Autodesk Inventor part; units mm, degrees
sketch "Sketch1" plane through (0, 0, 0) normal (0, 1, 0) x (-1, 0, 0)
  circle A0 centre (0, 0) radius 68.75
  dimension "d0" = 137.5
extrude "Extrusion1" add sketch "Sketch1" along normal blind 27.5
sketch "Sketch2" plane through (0, 27.5, 0) normal (0, 1, 0) x (1, 0, 0)
  circle A0 centre (0, 0) radius 66
  dimension "d4" = 132
extrude "Extrusion2" cut sketch "Sketch2" against normal blind 22.5
sketch "Sketch3" plane through (0, 5, 0) normal (0, 1, 0) x (1, 0, 0)
  circle A0 centre (0, 0) radius 68.75
  line L0 (0, 68.75) -> (0, 41.75)
  arc A1 (7.1286, 29.4112) -> (-7.3714, 29.5547) centre (0, 41.75) ccw
  line L1 (8.5358, 25.4622) -> (-8.9642, 25.4622)
  line L2 (8.5358, 25.4622) -> (8.5358, 28.5136)
  line L3 (-8.9642, 25.4622) -> (-8.9642, 28.7999)
  line L4 (-7.3714, 29.5547) -> (-7.3714, 27.0547)
  line L5 (-7.3714, 27.0547) -> (7.1286, 27.0547)
  line L6 (7.1286, 27.0547) -> (7.1286, 29.4112)
  arc A2 (19.25, 38.25) -> (19.25, 45.25) centre (19.25, 41.75) ccw
  line L7 (19.25, 45.25) -> (15.3562, 45.25)
  line L8 (19.25, 38.25) -> (15.3562, 38.25)
  arc A3 (-19.25, 45.25) -> (-19.25, 38.25) centre (-19.25, 41.75) ccw
  line L9 (-19.25, 45.25) -> (-15.3562, 45.25)
  line L10 (-19.25, 38.25) -> (-15.3562, 38.25)
  arc A4 (-15.3562, 38.25) -> (-8.9642, 28.7999) centre (0, 41.75) ccw
  arc A5 (8.5358, 28.5136) -> (15.3562, 38.25) centre (0, 41.75) ccw
  arc A6 (15.3562, 45.25) -> (-15.3562, 45.25) centre (0, 41.75) ccw
  dimension "d7" = 27
  dimension "d8" = 28.5
  dimension "d12" = 17.5
  dimension "d14" = 2.5
  dimension "d15" = 14.5
extrude "Extrusion3" add sketch "Sketch3" along normal blind 19.5 contours A6 L7 A2 L8 A5 L2 L1 L3 A4 L10 A3 L9
sketch "Sketch4" plane through (0, 24.5, 0) normal (0, 1, 0) x (1, 0, 0)
  line L0 (-8.9642, 25.4622) -> (8.5358, 25.4622)
  line L1 (-0.002, 25.4622) -> (2.998, 25.4622)
  line L2 (2.998, 25.4622) -> (2.998, 27.0547)
  line L3 (2.998, 27.0547) -> (-3.002, 27.0547)
  line L4 (7.1286, 27.0547) -> (-7.3714, 27.0547)
  line L5 (-3.002, 27.0547) -> (-3.002, 25.4622)
  line L6 (-3.002, 25.4622) -> (-0.002, 25.4622)
  point P0 (0, 0)
  dimension "d18" = 3
  dimension "d19" = 6
extrude "Extrusion4" cut sketch "Sketch4" against normal blind 4
sketch "Sketch5" plane through (0, 24.5, 0) normal (0, 1, 0) x (1, 0, 0)
  arc A0 (-19.25, 45.25) -> (-19.25, 38.25) centre (-19.25, 41.75) ccw
  circle A1 centre (-19.25, 41.75) radius 2
  arc A2 (19.25, 38.25) -> (19.25, 45.25) centre (19.25, 41.75) ccw
  circle A3 centre (19.25, 41.75) radius 2
  point P0 (0, 0)
  dimension "d24" = 4
  dimension "d25" = 4
extrude "Extrusion5" cut sketch "Sketch5" against normal blind 19
sketch "Sketch6" plane through (0, 5, 0) normal (0, 1, 0) x (1, 0, 0)
  line L0 (-30, 0) -> (-30, 17.25)
  line L1 (-30, 17.25) -> (-62, 17.25)
  line L2 (-62, 17.25) -> (-62, -17.25)
  line L3 (-62, -17.25) -> (-30, -17.25)
  line L4 (-30, -17.25) -> (-30, 0)
  point P0 (0, 0)
  dimension "d28" = 30
  dimension "d29" = 17.25
  dimension "d30" = 32
  dimension "d31" = 90
  dimension "d32" = 34.5
extrude "Extrusion6" cut sketch "Sketch6" against normal blind 2.75
sketch "Sketch7" plane through (0, 5, 0) normal (0, 1, 0) x (1, 0, 0)
  line L0 (-30, 17.25) -> (-30, -17.25)
  line L1 (-30, 0) -> (-26.25, 0)
  line L2 (-26.25, 0) -> (-26.25, 10.5)
  line L3 (-26.25, 10.5) -> (-26.25, -10.5) construction
  line L4 (-22.5, 6.75) -> (-22.5, -6.75)
  line L5 (-30, -6.75) -> (-30, 6.75)
  arc A0 (-22.5, 6.75) -> (-30, 6.75) centre (-26.25, 6.75) ccw
  arc A1 (-30, -6.75) -> (-22.5, -6.75) centre (-26.25, -6.75) ccw
  line L6 (-26.25, 0) -> (36.25, 0)
  line L7 (36.25, 0) -> (36.25, 10.5)
  line L8 (36.25, 10.5) -> (36.25, -10.5) construction
  line L9 (32.5, 6.75) -> (32.5, -6.75)
  line L10 (40, -6.75) -> (40, 6.75)
  arc A2 (40, 6.75) -> (32.5, 6.75) centre (36.25, 6.75) ccw
  arc A3 (32.5, -6.75) -> (40, -6.75) centre (36.25, -6.75) ccw
  line L11 (36.25, 10.5) -> (57.25, 10.5) construction
  point P0 (0, 0)
  dimension "d36" = 3.75
  dimension "d37" = 10.5
  dimension "d38" = 21
  dimension "d39" = 62.5
  dimension "d40" = 10.5
  dimension "d41" = 21
  dimension "d42" = 90
  dimension "d43" = 7.5
extrude "Extrusion7" add sketch "Sketch7" along normal blind 18
sketch "Sketch8" plane through (0, 5, 0) normal (0, 1, 0) x (1, 0, 0)
  line L0 (-22.5, 6.75) -> (-22.5, -6.75)
  line L1 (-22.5, 0) -> (-22.5, 10.5)
  line L2 (-22.5, 10.5) -> (31.5, 10.5)
  line L3 (31.5, 10.5) -> (31.5, -58.1)
  line L4 (31.5, -58.1) -> (-22.5, -58.1)
  line L5 (-22.5, -58.1) -> (-22.5, 10.5)
  point P0 (0, 0)
  dimension "d46" = 10.5
  dimension "d47" = 54
  dimension "d48" = 68.6
extrude "Extrusion8" cut sketch "Sketch8" against normal blind 3
ref_plane "Work Plane1" through (-22.5, 2, 58.1) normal (0, 0, -1) x (-1, 0, 0)
sketch "Sketch9" plane through (-22.5, 2, 58.1) normal (0, 0, -1) x (-1, 0, 0)
  line L0 (-53.8112, 3) -> (0, 3)
  line L1 (0, 3) -> (-9, 3)
  line L2 (-9, 3) -> (-9, 15)
  line L3 (-9, 15) -> (-21.5, 15)
  line L4 (-21.5, 15) -> (-21.5, 3)
  line L5 (-21.5, 3) -> (-9, 3)
  line L6 (-54, 0) -> (0, 0)
  point P0 (-22.5, -2)
  dimension "d52" = 12
  dimension "d53" = 12.5
extrude "Extrusion9" cut sketch "Sketch9" against normal blind 102
ref_plane "Work Plane2" through (68.75, 0, 0) normal (1, 0, 0) x (0, 1, 0)
sketch "Sketch10" plane through (68.75, 0, 0) normal (1, 0, 0) x (0, 1, 0)
  line L0 (0, -68.75) -> (0, 68.75)
  line L1 (0, 0) -> (2, 0)
  line L2 (1.5818, 0) -> (1.5818, -10)
  line L3 (1.5818, -10) -> (21.5818, -10)
  line L4 (21.5818, -10) -> (21.5818, 10)
  line L5 (5, 10.5) -> (23, 10.5)
  line L6 (21.5818, 10) -> (1.5818, 10)
  line L7 (1.5818, 10) -> (1.5818, 0)
  line L8 (2, -10.5) -> (2, 58.1)
  point P0 (2, 10)
  point P1 (2, -10)
  dimension "d64" = 10
  dimension "d65" = 20
  dimension "d66" = 20
  dimension "d67" = 20
extrude "Extrusion10" cut sketch "Sketch10" against normal blind 5 contours L8 L6 L4 L3
sketch "Sketch11" plane through (0, 23, 0) normal (0, 1, 0) x (1, 0, 0)
  arc A0 (40, 6.75) -> (32.5, 6.75) centre (36.25, 6.75) ccw
  circle A1 centre (36.25, 6.75) radius 2
  arc A2 (32.5, -6.75) -> (40, -6.75) centre (36.25, -6.75) ccw
  circle A3 centre (36.25, -6.75) radius 2
  arc A4 (-22.5, 6.75) -> (-30, 6.75) centre (-26.25, 6.75) ccw
  circle A5 centre (-26.25, 6.75) radius 2
  arc A6 (-30, -6.75) -> (-22.5, -6.75) centre (-26.25, -6.75) ccw
  circle A7 centre (-26.25, -6.75) radius 2
  point P0 (0, 0)
  dimension "d70" = 4
  dimension "d71" = 4
  dimension "d72" = 4
  dimension "d73" = 4
extrude "Extrusion11" cut sketch "Sketch11" against normal blind 12
properties part number "gehäuse_scan"
Geometry check sheet. Reference: the model listing, model coordinates, mm. A direction names the side the tool comes from. Give positions to 0.01 mm unless a question says otherwise; leave off trailing zeros. Loops run counter-clockwise (first coordinate to the right, second up) from the corner with the lowest first, then second, coordinate; pieces in that order, holes last. Notation, with made-up numbers: (57.25, 72.5) - (85.25, 72.5) arc R21 ccw to (85.25, 95.5) - close; hole circle Ø10 at (66.25, -1). An arc over 180 degrees is marked (long way). Use CSV: the item, a comma, the result in double quotes. Start each with the question number.
Q1. Access from +Z, -Z, +X, -X, +Y, -Y to the whole of each face (thin tool, end or side, straight path). Record for faces 3 (the face through (36.3, 13.9, 10.5)), 4 (the face through (1, 0, 1)).
Q2. Scan lines: probe 1 along X at (y, z) = (12, 0); probe 2 along X at (y, z) = (18, -6.75); probe 3 along Z at (x, y) = (-26.25, 20). Record each from-to range of solid material in increasing order. Write a range as from..to.
Q3. Release check for a two-part mould opening along X. For faces 1 (the face through (66, 2, 0)), 2 (the face through (-24.342, 17.084, -7.351)) record: +X half, -X half, draft (parallel to the pull), parting line (faces both ways), or undercut.
Q4. Go/stop test with flat-tipped pins: pin 1 Ø1.9 at (y, z) = (10.5, -28.5) entering from -X; pin 2 Ø1.5 at (y, z) = (21, 4) entering from +X; pin 3 Ø1.2 at (x, z) = (37, -6) entering from +Y. Record where each tip stops, or that it passes through.
Q5. Section check B-B, the plane x = -26.25. Record the cut outline in (y, z), and give its area (3 significant figures).
Q6. Section check D-D, the plane z = 60. Record the cut outline in (x, y), and give its area (3 significant figures).
Q7. Section check C-C, the plane z = -41.75. Record the cut outline in (x, y).
Q8. Section check A-A, the plane z = 0. Record the cut outline in (x, y).
Findings below:
1,face 3,"+Y"
1,face 4,"+Z, -Z, +X, -X, -Y"
2,probe 1,"x = -68.75..-66, -30..-22.5, 32.5..40"
2,probe 2,"x = -68.42..-65.65, -30..-28.25, -24.25..-22.5, 32.5..34.25, 38.25..40"
2,probe 3,"z = -63.54..-60.56, -10.5..-8.75, -4.75..4.75, 8.75..10.5, 60.56..63.54"
3,face 1,"draft"
3,face 2,"undercut"
4,pin 1,"stops at x = -62.99"
4,pin 2,"stops at x = 68.66"
4,pin 3,"stops at y = 11"
5,outline,"(0, -63.54) - (27.5, -63.54) - (27.5, -60.56) - (5, -60.56) - (5, -10.5) - (23, -10.5) - (23, -8.75) - (11, -8.75) - (11, -4.75) - (23, -4.75) - (23, 4.75) - (11, 4.75) - (11, 8.75) - (23, 8.75) - (23, 10.5) - (5, 10.5) - (5, 60.56) - (27.5, 60.56) - (27.5, 63.54) - (0, 63.54) - close"
5,area,"1,050 mm^2"
6,outline,"(-33.56, 0) - (33.56, 0) - (33.56, 27.5) - (27.5, 27.5) - (27.5, 5) - (-27.5, 5) - (-27.5, 27.5) - (-33.56, 27.5) - close"
6,area,"609 mm^2"
7,outline,"(-54.62, 0) - (54.62, 0) - (54.62, 27.5) - (51.12, 27.5) - (51.12, 5) - (22.75, 5) - (22.75, 24.5) - (21.25, 24.5) - (21.25, 5.5) - (17.25, 5.5) - (17.25, 24.5) - (14.25, 24.5) - (14.25, 5) - (-14.25, 5) - (-14.25, 24.5) - (-17.25, 24.5) - (-17.25, 5.5) - (-21.25, 5.5) - (-21.25, 24.5) - (-22.75, 24.5) - (-22.75, 5) - (-51.12, 5) - (-51.12, 27.5) - (-54.62, 27.5) - close"
8,outline,"(-68.75, 0) - (68.75, 0) - (68.75, 2) - (63.75, 2) - (63.75, 5) - (40, 5) - (40, 23) - (32.5, 23) - (32.5, 5) - (31.5, 5) - (31.5, 2) - (-22.5, 2) - (-22.5, 23) - (-30, 23) - (-30, 2.25) - (-62, 2.25) - (-62, 5) - (-66, 5) - (-66, 27.5) - (-68.75, 27.5) - close; (66, 21.58) - (68.75, 21.58) - (68.75, 27.5) - (66, 27.5) - close"
